Autodesk Fusion 360 part; units mm, degrees
sketch "Sketch1" plane through (0, 0, 0) normal (0, 1, 0) x (1, 0, 0)
  circle A0 centre (0, 0) radius 11
  circle A1 centre (0, 0) radius 7.5
  dimension "d1" = 22
  dimension "d2" = 15
ref_plane "WorkPlane1" through (0, 138, 0) normal (0, 1, 0) x (1, 0, 0)
ref_plane "WorkPlane2" through (0, -20, 0) normal (0, 1, 0) x (1, 0, 0)
sketch "Sketch2" plane through (0, -20, 0) normal (0, 1, 0) x (1, 0, 0)
  circle A0 centre (0, 0) radius 7.5
  circle A1 centre (0, 0) radius 10.5
  dimension "d5" = 21
sketch "Sketch3" plane through (0, 138, 0) normal (0, 1, 0) x (1, 0, 0)
  circle A0 centre (0, 0) radius 7.5
  circle A1 centre (0, 0) radius 11
  line L0 (0, 0) -> (20, 0) construction
  line L1 (-12, 0) -> (13, 0)
  line L2 (-11.2763, -4.1042) -> (12.216, 4.4463)
  line L3 (-9.1925, -7.7135) -> (9.9586, 8.3562)
  line L4 (-6, -10.3923) -> (6.5, 11.2583)
  line L5 (-2.0838, -11.8177) -> (2.2574, 12.8025)
  line L6 (2.0838, -11.8177) -> (-2.2574, 12.8025)
  line L7 (6, -10.3923) -> (-6.5, 11.2583)
  line L8 (9.1925, -7.7135) -> (-9.9586, 8.3562)
  line L9 (11.2763, -4.1042) -> (-12.216, 4.4463)
ref_plane "WorkPlane3" through (0, 148, 0) normal (0, 1, 0) x (1, 0, 0)
sketch "Sketch4" plane through (0, 148, 0) normal (0, 1, 0) x (1, 0, 0)
  circle A0 centre (0, 0) radius 7.5
  circle A1 centre (0, 0) radius 14
  dimension "d10" = 28
extrude "Extrude1" add sketch "Sketch4" along normal blind 2 contours A0 | A1 makes body 1
loft "Loft1" add profiles "Sketch2", "Sketch1", "Sketch3" section 1 section 2 section 3 contours A0 A1 L1 L9 | A0 A1 L1 L2 | A0 A1 L2 L3 | A0 A1 L8 L9 | A0 A1 L3 L4 | A0 A1 L7 L8 | A0 A1 L1 L9 | A0 A1 L1 L2 | A0 A1 L2 L3 | A0 A1 L3 L4 | A0 A1 L4 L5 | A0 A1 L4 L5 | A0 A1 L5 L6 | A0 A1 L5 L6 | A0 A1 L6 L7 | A0 A1 L6 L7 | A0 A1 L7 L8 | A0 A1 L8 L9 separate body makes body 2
extrude "Extrude2" cut sketch "Sketch2" along normal blind 160 contours A0 bodies 2
extrude "Extrude3" add sketch "Sketch3" along normal blind 10 contours A0 A1 L1 L9 | A0 A1 L2 L3 | A0 A1 L7 L8 | A0 A1 L1 L2 | A0 A1 L3 L4 | A0 A1 L4 L5 | A0 A1 L5 L6 | A0 A1 L6 L7 | A0 A1 L8 L9 picked at (9.446, -2.6762) picked at (9.0714, 3.7547) picked at (6.4214, -7.4266) picked at (-9.8085, -0.4257) picked at (-6.1987, -7.6135) picked at (2.1224, 9.5856) picked at (-0.1454, -9.8167) picked at (-4.5356, 8.7073) picked at (-9.0714, 3.7547) bodies 1 2
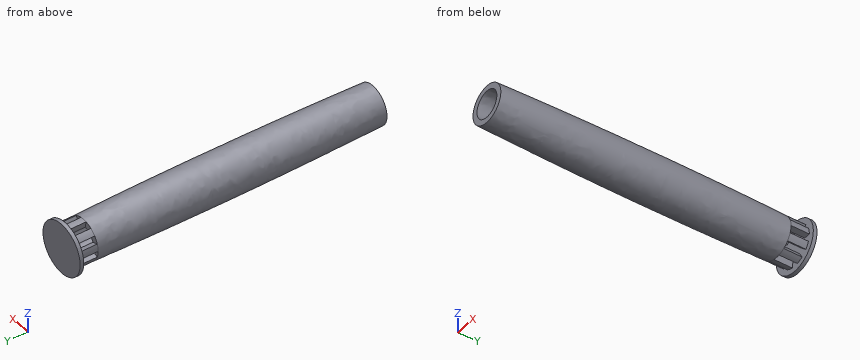
The listing builds one solid part. Answer for the finished solid, in the listing's coordinates (mm). Give positions to 0.01 mm unless a question says otherwise; leave off trailing zeros. Answer as a JSON object with one key per item and string values. Group by question number.
Item 1: Flat-ended cylindrical pins translate along their axes: pin 1 (3 mm diameter, centred on x = 9, y = 144.5, fed in from -Z); pin 2 (5 mm diameter, centred on x = -11, z = 9.5, fed in from -Y); pin 3 (12 mm diameter, centred on y = 101.5, z = -9.5, fed in from -X); pin 4 (8 mm diameter, centred on x = 11, z = -6, fed in from -Y). Find the tip coordinate at first contact, or state that the pin passes through.
Item 2: Consider L1, parallel to Z at x = 0.5, y = 70; L2, parallel to Y at x = 7.5, z = 3.5; L3, parallel to X at y = 65, z = 0. Determine where each line is inside the solid, lowest interval first. Write a range as from..to.
Item 3: The part is cut by section A-A on y = 139.5. Give the number of separate pieces and of enclosed holes in the cut face, and give its area (3 significant figures).
Result set:
{
 "1": {"pin 1": "z = -7.07", "pin 2": "y = 148", "pin 3": "x = -11.05", "pin 4": "y = -20"},
 "2": {"L1": "-11.74..-7.48, 7.48..11.74", "L2": "-20..138, 148..150", "L3": "-11.75..-7.5, 7.5..11.75"},
 "3": {"separate pieces": "9", "enclosed holes": "0", "area": "102 mm²"}
}
